```python
from build123d import *

# Parameters (mm, degrees)
SKETCH_1_R          = 5
SKETCH_1_R_2        = 3
EXTRUDE_1_DEPTH     = 7.5
SKETCH_2_R          = 3.6
CUT_EXTRUDE_1_DEPTH = 2
SKETCH_3_R          = 2.9
EXTRUDE_2_DEPTH     = 3
FILLET_1_R          = 2
SKETCH_4_R          = 2.9
EXTRUDE_3_DEPTH     = 10
FILLET_2_R          = 2.9
FILLET_3_R          = 3


with BuildPart() as part:
    # 스케치1 → 보스-돌출1 (new body)
    # profile 1 of 5: a face of its own
    with BuildSketch(Plane.XY):
        with BuildLine():
            Line((8.866410343, 21.94338903), (4.384187039, 21.94338903))
            Line((4.384187039, 21.94338903), (2.987768149, 19.65002342))
            Line((2.987768149, 19.65002342), (2.987768149, 17.661246793))
            Line((2.987768149, 17.661246793), (2.987768149, 9.70876495))
            Line((2.987768149, 9.70876495), (-3.184671245, 3.854590647))
            ThreePointArc((-3.184671245, 3.854590647), (2.13033375, 4.523458645), (5, 0))
            ThreePointArc((5, 0), (0, -5), (-5, 0))
            Line((-5, 0), (-5, -10.071407464))
            Line((-5, -10.071407464), (-16.264805165, -9.728236855))
            Line((-16.264805165, -9.728236855), (-17.766639728, -13.42657959))
            Line((-17.766639728, -13.42657959), (-19.940502755, -13.22881584))
            ThreePointArc((-19.940502755, -13.22881584), (-21.568981751, -13.840235901), (-22.102673306, -15.49581787))
            ThreePointArc((-22.102673306, -15.49581787), (-21.54079944, -16.765444299), (-20.287735083, -17.363343312))
            Line((-20.287735083, -17.363343312), (-13.716958703, -17.9611093))
            ThreePointArc((-13.716958703, -17.9611093), (-10.295562947, -19.77999502), (-9.201017746, -23.497018692))
            Line((-9.201017746, -23.497018692), (-13.218080179, -30.193463728))
            ThreePointArc((-13.218080179, -30.193463728), (-13.817495958, -30.9099569), (-14.608237914, -31.407338947))
            Line((-14.608237914, -31.407338947), (-15.680360182, -31.867141901))
            ThreePointArc((-15.680360182, -31.867141901), (-17.282818205, -32.73507756), (-18.70115036, -33.879419256))
            Line((-18.70115036, -33.879419256), (-21.587390027, -36.678865361))
            ThreePointArc((-21.587390027, -36.678865361), (-23.484754079, -39.219572782), (-24.491261067, -42.226585957))
            ThreePointArc((-24.491261067, -42.226585957), (-23.966473892, -51.146683639), (-19.652431958, -58.971808969))
            ThreePointArc((-19.652431958, -58.971808969), (-17.283591849, -59.850561763), (-15.231880476, -58.376082064))
            ThreePointArc((-15.231880476, -58.376082064), (-15.139015744, -57.789610004), (-15.395055283, -57.253870245))
            ThreePointArc((-15.395055283, -57.253870245), (-18.621303847, -45.462540141), (-11.334185384, -35.647141528))
            ThreePointArc((-11.334185384, -35.647141528), (-10.571184727, -35.206851872), (-9.849893086, -34.701121359))
            ThreePointArc((-9.849893086, -34.701121359), (-8.133553397, -33.471894478), (-6.337557558, -32.362291125))
            ThreePointArc((-6.337557558, -32.362291125), (-5.290911527, -31.673468731), (-4.338619501, -30.85916897))
            Line((-4.338619501, -30.85916897), (6.238088337, -20.600518625))
            Line((6.238088337, -20.600518625), (8.3701186, -14.978169718))
            ThreePointArc((8.3701186, -14.978169718), (8.662275884, -14.729272874), (8.69193724, -14.346616734))
            ThreePointArc((8.69193724, -14.346616734), (8.365752146, -12.021808556), (8.866410343, -9.728236855))
            Line((8.866410343, -9.728236855), (8.866410343, 21.94338903))
        make_face()
    # profile 2 of 5: a face of its own
    with BuildSketch(Plane.XY):
        Circle(SKETCH_1_R)
        Circle(SKETCH_1_R_2, mode=Mode.SUBTRACT)
    # profile 3 of 5: a face of its own
    with BuildSketch(Plane.XY):
        with BuildLine():
            ThreePointArc((5, 0), (2.13033375, 4.523458645), (-3.184671245, 3.854590647))
            ThreePointArc((-3.184671245, 3.854590647), (-4.523458645, 2.13033375), (-5, 0))
            ThreePointArc((-5, 0), (0, -5), (5, 0))
        make_face()
        Circle(SKETCH_1_R_2, mode=Mode.SUBTRACT)
    # profile 4 of 5: a face of its own
    with BuildSketch(Plane.XY):
        Polygon((8.866410343, 25.078081763), (7.518879772, 25.078081763), (4.384187039, 21.94338903), (8.866410343, 21.94338903), align=None)
    # profile 5 of 5: a face of its own
    with BuildSketch(Plane.XY):
        with BuildLine():
            Line((8.866410343, 21.94338903), (4.384187039, 21.94338903))
            Line((4.384187039, 21.94338903), (2.987768149, 19.65002342))
            Line((2.987768149, 19.65002342), (2.987768149, 17.661246793))
            Line((2.987768149, 17.661246793), (2.987768149, 9.70876495))
            Line((2.987768149, 9.70876495), (-3.184671245, 3.854590647))
            ThreePointArc((-3.184671245, 3.854590647), (2.13033375, 4.523458645), (5, 0))
            ThreePointArc((5, 0), (0, -5), (-5, 0))
            Line((-5, 0), (-5, -10.071407464))
            Line((-5, -10.071407464), (-16.264805165, -9.728236855))
            Line((-16.264805165, -9.728236855), (-17.766639728, -13.42657959))
            Line((-17.766639728, -13.42657959), (-19.940502755, -13.22881584))
            ThreePointArc((-19.940502755, -13.22881584), (-21.568981751, -13.840235901), (-22.102673306, -15.49581787))
            ThreePointArc((-22.102673306, -15.49581787), (-21.54079944, -16.765444299), (-20.287735083, -17.363343312))
            Line((-20.287735083, -17.363343312), (-13.716958703, -17.9611093))
            ThreePointArc((-13.716958703, -17.9611093), (-10.295562947, -19.77999502), (-9.201017746, -23.497018692))
            Line((-9.201017746, -23.497018692), (-13.218080179, -30.193463728))
            ThreePointArc((-13.218080179, -30.193463728), (-13.817495958, -30.9099569), (-14.608237914, -31.407338947))
            Line((-14.608237914, -31.407338947), (-15.680360182, -31.867141901))
            ThreePointArc((-15.680360182, -31.867141901), (-17.282818205, -32.73507756), (-18.70115036, -33.879419256))
            Line((-18.70115036, -33.879419256), (-21.587390027, -36.678865361))
            ThreePointArc((-21.587390027, -36.678865361), (-23.484754079, -39.219572782), (-24.491261067, -42.226585957))
            ThreePointArc((-24.491261067, -42.226585957), (-23.966473892, -51.146683639), (-19.652431958, -58.971808969))
            ThreePointArc((-19.652431958, -58.971808969), (-17.283591849, -59.850561763), (-15.231880476, -58.376082064))
            ThreePointArc((-15.231880476, -58.376082064), (-15.139015744, -57.789610004), (-15.395055283, -57.253870245))
            ThreePointArc((-15.395055283, -57.253870245), (-18.621303847, -45.462540141), (-11.334185384, -35.647141528))
            ThreePointArc((-11.334185384, -35.647141528), (-10.571184727, -35.206851872), (-9.849893086, -34.701121359))
            ThreePointArc((-9.849893086, -34.701121359), (-8.133553397, -33.471894478), (-6.337557558, -32.362291125))
            ThreePointArc((-6.337557558, -32.362291125), (-5.290911527, -31.673468731), (-4.338619501, -30.85916897))
            Line((-4.338619501, -30.85916897), (6.238088337, -20.600518625))
            Line((6.238088337, -20.600518625), (8.3701186, -14.978169718))
            ThreePointArc((8.3701186, -14.978169718), (8.662275884, -14.729272874), (8.69193724, -14.346616734))
            ThreePointArc((8.69193724, -14.346616734), (8.365752146, -12.021808556), (8.866410343, -9.728236855))
            Line((8.866410343, -9.728236855), (8.866410343, 21.94338903))
        make_face()
    extrude(amount=EXTRUDE_1_DEPTH)

    # 스케치2 → 컷-돌출1 (cut)
    with BuildSketch(Plane(origin=(8.866410343, 0, 0), x_dir=(0, 0, -1), z_dir=(1, 0, 0))):
        with Locations(Location((-3.75, 15.078081763, 0), (0, 0, 90))):
            Circle(SKETCH_2_R)
    extrude(amount=-CUT_EXTRUDE_1_DEPTH, mode=Mode.SUBTRACT)

    # 스케치3 → 보스-돌출2 (add)
    with BuildSketch(Plane(origin=(6.866410343, 0, 0), x_dir=(0, 0, -1), z_dir=(1, 0, 0))):
        with Locations(Location((-3.75, 15.078081763, 0), (0, 0, 90))):
            Circle(SKETCH_3_R)
    extrude(amount=EXTRUDE_2_DEPTH)

    # 필렛1
    fillet_1_edges = [part.edges().sort_by_distance(p)[0] for p in [
        (9.866410343, 12.178081763, 3.75),
    ]]
    fillet(fillet_1_edges, radius=FILLET_1_R)

    # 스케치4 → 보스-돌출3 (add)
    with BuildSketch(Plane(origin=(-1.357268469, -14.919396185, 0), x_dir=(0.995887428286197, -0.09059928355955607, 0), z_dir=(0.09059928355955607, 0.995887428286197, 0))):
        with Locations(Location((-11.657618139, -3.8, 0), (0, 0, 180))):
            Circle(SKETCH_4_R)
    extrude(amount=EXTRUDE_3_DEPTH)

    # 필렛2
    fillet_2_edges = [part.edges().sort_by_distance(p)[0] for p in [
        (-9.17287744, -4.167087973, 3.8),
    ]]
    fillet(fillet_2_edges, radius=FILLET_2_R)

    # 필렛3
    fillet_3_edges = [part.edges().sort_by_distance(p)[0] for p in [
        (-5, -10.071407464, 3.75),
    ]]
    fillet(fillet_3_edges, radius=FILLET_3_R)


solid = part.part
```
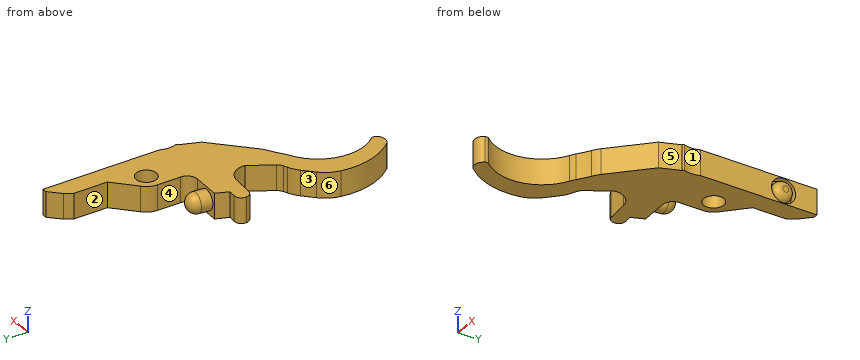
CAD build for the part. Positions are in the model's coordinates, mm. Face numbers are marked on the shaded views. A direction names the side the tool comes from. Round coordinates to 2 decimals unless told otherwise and drop trailing zeros. Write each loop counter-clockwise with the first axis right and the second up, starting at its lowest first coordinate (ties: lowest second). Pieces come first, ordered by that corner, then holes. Notation, with made-up numbers: (64.25, 8) -> (110.25, 8) arc R23 cw to (110.25, 19) -> close; hole circle Ø9 at (-11.75, 28.5). An arc over 180 degrees is marked (long way). Answer in a Markdown table with one row per item. Add a question column.
Item 1: Saw through at B-B, the plane y = 6. Write the cut outline in (x, z).
Item 2: Drop flat-ended pins along their axis: pin 1 Ø2 at (y, z) = (-34, 3.5) entering from -X; pin 2 Ø2 at (x, y) = (3.5, -21) entering from -Z; pin 3 Ø1.5 at (y, z) = (-23.5, 5) entering from -X; pin 4 Ø1.5 at (y, z) = (-10.5, 1.5) entering from -X. Give the stop position or say it passes through.
Item 3: Mould opens along X. For the marked faces 4, 5 and 6 say: pulls with the +X half, pulls with the -X half, needs draft (parallel to the pull), parting line crosses it, or undercut.
Item 4: Drill centre lines: line 1 (Y direction, x = -16.5, z = 5.5); line 2 (Y direction, x = 0, z = 3.75); line 3 (X direction, y = -1, z = 1.5). Where is each one in solid material? Low to high. Write a range as from..to.
Item 5: Saw through at A-A, the plane x = 0. Write the cut outline in (y, z), then the cut area to 3 significant figures.
Item 6: Which spindle directions (+Z, -Z, +X, -X, +Y, -Y) get a long thin tool onto all of the face, cutting with end or side? Do the marked faces 1, 2 and 3. Say none if no direction does.
Item 7: Saw through at C-C, the plane y = -44.5. Write the cut outline in (x, z).
Findings below:
| question | item | result |
|---|---|---|
| 1 | outline | (-0.92, 0) -> (8.87, 0) -> (8.87, 7.5) -> (-0.92, 7.5) -> close |
| 2 | pin 1 | stops at x = -19.86 |
| 2 | pin 2 | stops at z = 0 |
| 2 | pin 3 | stops at x = -9.65 |
| 2 | pin 4 | stops at x = -16.88 |
| 3 | face 4 | undercut |
| 3 | face 5 | pulls with the +X half |
| 3 | face 6 | pulls with the -X half |
| 4 | line 1 | y = -59.62..-55.82, -40.27..-32.26, -17.71..-10.31 |
| 4 | line 2 | y = -26.65..-3, 3..6.88 |
| 4 | line 3 | x = -5..-2.83, 2.83..8.87 |
| 5 | outline | (-26.65, 0) -> (-3, 0) -> (-3, 7.5) -> (-26.65, 7.5) -> close; (3, 0) -> (6.88, 0) -> (6.88, 7.5) -> (3, 7.5) -> close |
| 5 | area | 206 mm^2 |
| 6 | face 1 | +Z, -Z, +X |
| 6 | face 2 | +Z, -Z, -X, +Y |
| 6 | face 3 | +Z, -Z, -X |
| 7 | outline | (-24.74, 0) -> (-18.4, 0) -> (-18.4, 7.5) -> (-24.74, 7.5) -> close |
